```python
from build123d import *

# Parameters (mm, degrees)
F0_R        = 1
F1_DEPTH    = 1.2
F2_T1_DEPTH = 1.2
F3_R        = 5


# Not quite as in the source:
# - a fillet or chamfer that OpenCascade refuses, or shapes differently, is made with other operations: its cross-section is extruded or revolved along the edge and cut away or added


with BuildPart() as f1:
    # F0 (on Front) → F1 (new body)
    with BuildSketch(Plane.XZ):
        with BuildLine():
            ThreePointArc((-1, -11.9080854884), (0, 11.95), (1, -11.9080854884))
            Line((1, -11.9080854884), (1, -16.3193903072))
            ThreePointArc((1, -16.3193903072), (3.8276067146, -15.8956574837), (6.5381625357, -14.9858243236))
            Line((6.5381625357, -14.9858243236), (5.5446488339, -12.8552273145))
            ThreePointArc((5.5446488339, -12.8552273145), (0.2154334831, 14.9485032399), (-5.9128007498, -12.6901058819))
            Line((-5.9128007498, -12.6901058819), (-6.90530659, -14.8202307977))
            ThreePointArc((-6.90530659, -14.8202307977), (-4.0231005306, -15.8473077247), (-1, -16.3193903072))
            Line((-1, -16.3193903072), (-1, -11.9080854884))
        make_face()
        with Locations((-3.0301545951, -13.6681440997)):
            Circle(F0_R, mode=Mode.SUBTRACT)
        with Locations((3.0301545951, -13.6681440997)):
            Circle(F0_R, mode=Mode.SUBTRACT)
    extrude(amount=F1_DEPTH)

    # F2: fillet of radius 10 on 2 edges, made by hand

    # F2_s2 → F2_t1 (join)
    with BuildSketch(Plane.XZ):
        with BuildLine():
            ThreePointArc((-9.7709471746, -10.1486206785), (-8.0118480734, -12.2842810829), (-6.90530659, -14.8202307977))
            Line((-6.90530659, -14.8202307977), (-5.9128007498, -12.6901058819))
            ThreePointArc((-5.9128007498, -12.6901058819), (-7.9440740778, -11.5745099677), (-9.7709471746, -10.1486206785))
        make_face()
        with BuildLine():
            ThreePointArc((6.5381625357, -14.9858243236), (7.7071981674, -12.4786621044), (9.5183975603, -10.3877141232))
            ThreePointArc((9.5183975603, -10.3877141232), (7.6320006174, -11.7832822229), (5.5446488339, -12.8552273145))
            Line((5.5446488339, -12.8552273145), (6.5381625357, -14.9858243236))
        make_face()
    extrude(amount=F2_T1_DEPTH)

    # F3
    f3_edges = [f1.edges().sort_by_distance(p)[0] for p in [
        (-6.905307, -0.6, -14.820231),
        (6.538163, -0.6, -14.985824),
    ]]
    fillet(f3_edges, radius=F3_R)


solid = f1.part
```
The model under review builds one solid part; all positions refer to its coordinate system, in mm. A direction names the side the tool comes from. Coordinates: 2 decimals unless noted, no trailing zeros. Order: outer loops, then holes, each group sorted by start corner. A loop starts at its lowest first (then second) coordinate and runs counter-clockwise, first axis right, second up. Notation, with made-up numbers: (-9, 15.5) -> (17, 15.5) arc R20 cw to (17, 42.5) -> close; hole circle Ø2 at (-21, -21). An arc over 180 degrees is marked (long way). Answer in a Markdown table with one row per item. Add a question column.
Item 1: Clearance check with a flat-ended pin moving along its axis: pin 1 (1.2 mm diameter, centred on x = -3.03, z = -13.67, fed in from -Y). State where the tip first meets the part, or that it passes through.
Item 2: We need section B-B on z = -3.5. Write out the cut boundary in (x, y).
Item 3: We need section C-C on x = 0. Write out the cut boundary in (y, z), plus the area to 3 significant figures.
Item 4: Machinability: for faces 4 (the flat face through (-5.4, 0, 11)), 5 (the flat face through (-1, -1, -14)), which of the approach directions +Z, -Z, +X, -X, +Y, -Y give a long, thin tool a straight path to every point of the face, cutting with its end or side? Answer none if there is none.
Item 5: We need section A-A on x = 11.5. Write out the cut boundary in (y, z).
Item 6: To check wall thickness, follow probe 1 along Z at (x, y) = (-3.5, -0.5); probe 2 along Z at (x, y) = (2.75, -0.95); probe 3 along X at (y, z) = (-0.45, 7.5). State the ranges of each line that lie inside material, in increasing order.
Item 7: We need section D-D on y = -0.7. Give the number of separate pieces and of enclosed holes in the cut face, plus the area to 3 significant figures.
Item 8: Mouldability with a two-part tool opening along X and no side actions: class faces 1 (the flat face through (1, -1, -14)), 2 (the cylindrical face through (2.498, -0.592, -16.158)), 3 (the cylindrical face through (-2.74, -0.59, -16.12)) as +X half, -X half, draft (parallel to the pull), parting line (faces both ways), or undercut.
Final values:
| question | item | result |
|---|---|---|
| 1 | pin 1 | passes through |
| 2 | outline | (-13.88, -1.2) -> (-11.43, -1.2) -> (-11.43, 0) -> (-13.88, 0) -> close; (11.43, -1.2) -> (13.9, -1.2) -> (13.9, 0) -> (11.43, 0) -> close |
| 3 | outline | (-1.2, 11.95) -> (0, 11.95) -> (0, 14.95) -> (-1.2, 14.95) -> close |
| 3 | area | 3.60 mm2 |
| 4 | face 4 | +Z, -Z, +X, -X, +Y |
| 4 | face 5 | -Z, +Y, -Y |
| 5 | outline | (-1.2, -8.27) -> (0, -8.27) -> (0, -3.25) -> (-1.2, -3.25) -> close; (-1.2, 3.25) -> (0, 3.25) -> (0, 9.26) -> (-1.2, 9.26) -> close |
| 6 | probe 1 | z = -15.97 to -14.55, -12.79 to -11.43, 11.43 to 14.52 |
| 6 | probe 2 | z = -16.12 to -14.63, -12.71 to -11.63, 11.63 to 14.69 |
| 6 | probe 3 | x = -12.64 to -9.3, 9.3 to 12.65 |
| 7 | separate pieces | 1 |
| 7 | enclosed holes | 2 |
| 7 | area | 229 mm2 |
| 8 | face 1 | undercut |
| 8 | face 2 | +X half |
| 8 | face 3 | -X half |
